The listing builds one solid part. Answer for the finished solid, in the listing's coordinates (mm). A direction names the side the tool comes from. Give positions to 0.01 mm unless a question says otherwise; leave off trailing zeros. Order: outer loops, then holes, each group sorted by start corner. A loop starts at its lowest first (then second) coordinate and runs counter-clockwise, first axis right, second up. Notation, with made-up numbers: M 88,87.25 L 138,87.25 A13 ccw 138,103.25 Z; hole C 68.25,83 d7. An arc over 180 degrees is marked long. Answer as a JSON object with one key per item and string values. Group by question number.
Autodesk Inventor part; units mm, degrees
ref_plane "YZ Plane" through (0, 0, 0) normal (1, 0, 0) x (0, 1, 0)
ref_plane "XZ Plane" through (0, 0, 0) normal (0, 1, 0) x (-1, 0, 0)
ref_plane "XY Plane" through (0, 0, 0) normal (0, 0, 1) x (1, 0, 0)
sketch "Sketch1" plane through (0, 0, 0) normal (0, 0, 1) x (1, 0, 0)
  line L0 (0, 0) -> (-5, 0)
  line L1 (-5, 0) -> (-5, -43.15)
  line L2 (-5, -43.15) -> (0, -43.15)
  line L3 (0, -43.15) -> (0, 0)
  line L4 (0, 0) -> (-13.1356, 0) construction
  dimension "d1" = 43.15
  dimension "d2" = 5
revolve "Shoulder" add sketch "Sketch1" angle 360 about axis through (0, -43.15, 0) along (0, 1, 0)
sketch "Sketch2" plane through (0, 0, 0) normal (0, 1, 0) x (1, 0, 0)
  circle A0 centre (0, 0) radius 5
  circle A1 centre (0, 0) radius 4.76
  dimension "d3" = 9.52
extrude "Shoulder_neck" add sketch "Sketch2" along normal blind 1.85 contours A1
sketch "Sketch3" plane through (0, 1.85, 0) normal (0, 1, 0) x (1, 0, 0)
  circle A0 centre (0, 0) radius 4.76
  circle A1 centre (0, 0) radius 8.1
  dimension "d6" = 16.2
extrude "Head" add sketch "Sketch3" along normal blind 7 contours A0 | A1
sketch "Sketch4" plane through (0, -43.15, 0) normal (0, -1, 0) x (1, 0, 0)
  circle A0 centre (0, 0) radius 5
  circle A1 centre (0, 0) radius 3.09
  dimension "d9" = 6.18
extrude "Thread_neck" add sketch "Sketch4" along normal blind 2.6 contours A1
sketch "Sketch5" plane through (0, -45.75, 0) normal (0, -1, 0) x (1, 0, 0)
  circle A0 centre (0, 0) radius 3.09
  circle A1 centre (0, 0) radius 4
  dimension "d12" = 8
extrude "Thread_shoulder" add sketch "Sketch5" along normal blind 10.4 contours A0 | A1
sketch "Sketch6" plane through (0, 8.85, 0) normal (0, 1, 0) x (1, 0, 0)
  circle A0 centre (0, 0) radius 8.1
  circle A1 centre (0, 0) radius 2.5 construction
  line L0 (-2.5, 1.4434) -> (-2.5, -1.4434)
  line L1 (-2.5, -1.4434) -> (0, -2.8868)
  line L2 (0, -2.8868) -> (2.5, -1.4434)
  line L3 (2.5, -1.4434) -> (2.5, 1.4434)
  line L4 (2.5, 1.4434) -> (0, 2.8868)
  line L5 (0, 2.8868) -> (-2.5, 1.4434)
  dimension "d15" = 5
extrude "Hex" cut sketch "Sketch6" against normal blind 4.2 contours L5 L4 L3 L2 L1 L0
chamfer "Chamfer1" distance 0.24 angle 30 1 edges at (5, 0, 0) measured on face at (-4.8255, 0, -0.7786)
fillet "Fillet1" radius 0.4 1 edges at (-4.76, 1.85, 0)
chamfer "Chamfer2" distance 0.5 angle 30 1 edges at (-8.1, 8.85, 0) measured on face at (7.9951, 6.5167, 1.2993)
chamfer "Chamfer3" distance 0.625 angle 30 1 edges at (-4, -56.15, 0) measured on face at (0.7574, -56.15, 1.0973)
fillet "Fillet2" radius 0.7 1 edges at (-3.09, -43.15, 0)
chamfer "Chamfer7" distance 0.91 angle 30 1 edges at (-4, -45.75, 0) measured on face at (3.6579, -45.75, -0.3191)
thread "Thread"
equation "\"d3\" = Shoulder_neck_dia"
equation "\"d4\" = Shoulder_neck_length"
equation "\"d6\" = Head_diameter"
equation "\"d7\" = Head_height"
equation "\"d9\" = Thread_neck_dia"
equation "\"d10\" = Thread_neck_length"
equation "\"d12\" = Thread_diameter"
equation "\"d13\" = Thread_length - Thread_neck_length"
equation "\"d15\" = Hex_size"
equation "\"d16\" = Hex_length"
equation "\"d18\" = -0.5 * Shoulder_neck_dia + 0.5 * Shoulder_diameter"
equation "\"d64\" = -0.5 * Shoulder_neck_dia + 0.5 * Shoulder_diameter"
equation "\"d21\" = 0.1 * Hex_size"
equation "\"d65\" = 0.1 * Hex_size"
equation "\"d23\" = 0.5 * Thread_pitch"
equation "\"d66\" = 0.5 * Thread_pitch"
equation "\"d25\" = Thread_neck_radius"
equation "\"d60\" = -0.5 * Thread_neck_dia + 0.5 * Thread_diameter"
equation "\"d67\" = -0.5 * Thread_neck_dia + 0.5 * Thread_diameter"
equation "\"d1\" = Shoulder_length - Shoulder_neck_length"
equation "\"d2\" = 0.5 * Shoulder_diameter"
equation "\"Shoulder_length\" = 45"
equation "\"Shoulder_neck_dia\" = 9.52"
equation "\"Thread_diameter\" = 8"
equation "\"Thread_length\" = 13"
equation "\"Head_diameter\" = 16.2"
equation "\"Head_height\" = 7"
equation "\"Thread_neck_dia\" = 6.18"
equation "\"Hex_size\" = 5"
equation "\"Hex_length\" = 4.2"
equation "\"Thread_pitch\" = 1.25"
equation "\"Shoulder_neck_length\" = 1.85"
equation "\"Thread_neck_length\" = 2.6"
equation "\"Thread_neck_radius\" = 0.7"
properties part number "SCREW, SHOULDER, P, 12" material "Steel, High Strength Low Alloy"
Item 1: Section A-A (y = -49) is taken. Determine the outline of the cut face in (x, z).
Item 2: Consider probe 1 along Y at (x, z) = (6.75, 0); probe 2 along Z at (x, y) = (3.25, -34.5); probe 3 along Z at (x, y) = (3, -31). Determine where each line is inside the solid, lowest interval first. Write a range as from..to.
Item 3: A tool of negligible diameter and unlimited length cuts with its end or side. For faces 4 (the cylindrical face through (1.661, -44.787, -2.605)), 5 (the flat face through (0, 4.65, 0)), 6 (the cylindrical face through (-1.756, 5.054, -7.907)), 7 (the cylindrical face through (1.08, -21.95, 4.88)), from which of +Z, -Z, +X, -X, +Y, -Y can it reach the whole face along a straight path? Write none if from no direction.
Item 4: Flat-ended cylindrical pins translate along their axes: P1, Ø3, axis at y = -34, z = 1.5, coming from the +X side; P2, Ø5, axis at y = -1.5, z = -0.5, coming from the -X side; P3, Ø1, axis at y = -19.5, z = 1.5, coming from the -X side. Find the tip coordinate at first contact, or state that the pin passes through.
Item 5: Section B-B (y = -39) is taken. Determine the outline of the cut face in (x, z), and give its area (3 significant figures).
Item 6: Determine the mould class of faces 1 (the flat face through (-1.267, 6.779, 2.155)), 2 (the flat face through (-2, 8.85, -2)), 3 (the cylindrical face through (-0.867, -50.966, 3.905)) for opening direction Z: released by +Z, released by -Z, zero draft, split by the parting line, or undercut.
Values found:
{
 "1": {"outline": "C 0,0 d8"},
 "2": {"probe 1": "y = 1.85..8.85", "probe 2": "z = -3.8..3.8", "probe 3": "z = -4..4"},
 "3": {"face 4": "none", "face 5": "+Y", "face 6": "+Y, -Y", "face 7": "-Y"},
 "4": {"P1": "stops at x = 5", "P2": "stops at x = -5", "P3": "stops at x = -4.9"},
 "5": {"outline": "C 0,0 d10", "area": "78.5 mm^2"},
 "6": {"face 1": "undercut", "face 2": "zero draft", "face 3": "split by the parting line"}
}
